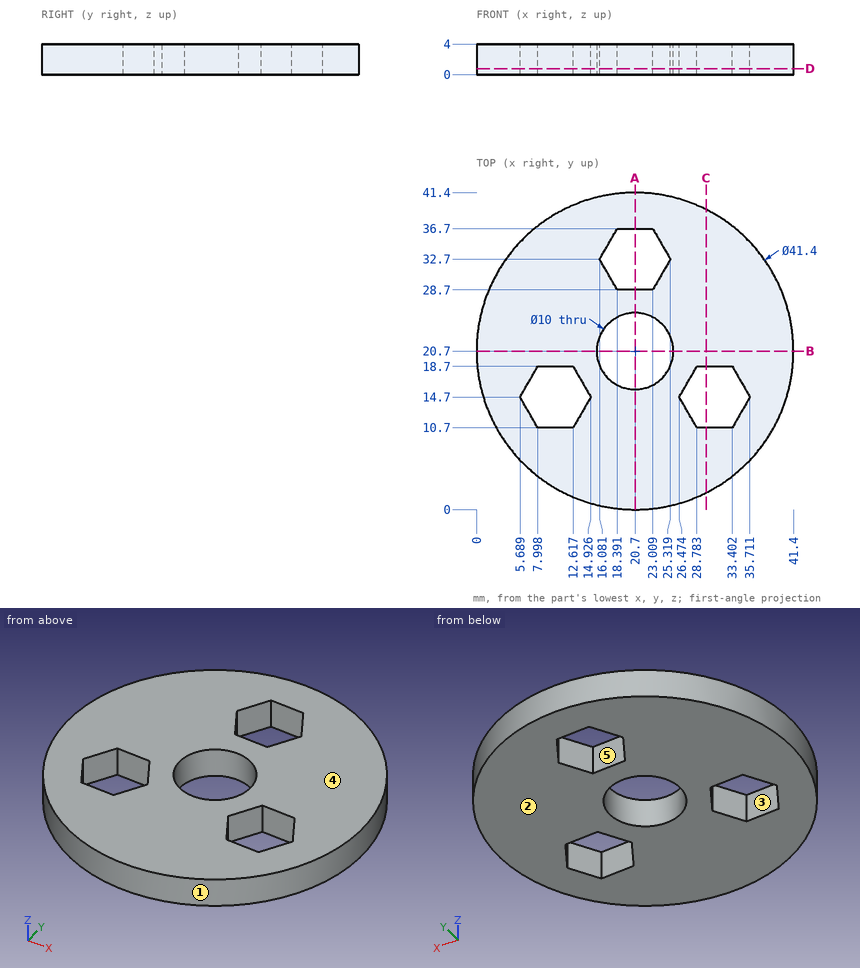
The drawing under review shows one solid part. Ordinate dimensions are in mm from its lowest x, y, z. A direction names the side the tool comes from. Coordinates: 2 decimals unless noted, no trailing zeros. Loops run counter-clockwise (first coordinate to the right, second up) from the corner with the lowest first, then second, coordinate; pieces in that order, holes last. Notation, with made-up numbers: (-36, 76) -> (4, 76) arc R13 cw to (4, 88) -> close; hole circle Ø11 at (24.5, 35). An arc over 180 degrees is marked (long way). Answer as a JSON object with one key per item and string values.
Q1. Take a section at B-B on y = 20.7. Give the boundary of the cut face in (x, z), plus the area to 3 significant figures.
Answer block:
{"outline": "(0, 0) -> (15.7, 0) -> (15.7, 4) -> (0, 4) -> close; (25.7, 0) -> (41.4, 0) -> (41.4, 4) -> (25.7, 4) -> close", "area": "126 mm^2"}
Q2. The part is to be moulded in two halves that separate along X. For the marked faces 1, 2 and 3, say which applies: +X half, -X half, draft (parallel to the pull), parting line (faces both ways), or undercut.
Answer block:
{"face 1": "parting line", "face 2": "draft", "face 3": "undercut"}
Q3. Tool access review of the marked faces 4 and 5: name each direction out of +Z, -Z, +X, -X, +Y, -Y from which nothing blocks a thin tool from reaching the whole face with its end or side.
Answer block:
{"face 4": "+Z, +X, -X, +Y, -Y", "face 5": "+Z, -Z"}
Q4. Take a section at A-A on x = 20.7. Give the boundary of the cut face in (y, z).
Answer block:
{"outline": "(0, 0) -> (15.7, 0) -> (15.7, 4) -> (0, 4) -> close; (25.7, 0) -> (28.7, 0) -> (28.7, 4) -> (25.7, 4) -> close; (36.7, 0) -> (41.4, 0) -> (41.4, 4) -> (36.7, 4) -> close"}
Q5. Clearance check with flat-ended pins moving along their axes: pin 1 Ø9 at (x, y) = (20.7, 20.7) entering from +Z; pin 2 Ø1 at (y, z) = (14.5, 2) entering from -X; pin 3 Ø1.5 at (y, z) = (14.5, 3.5) entering from +X; pin 4 Ø2 at (x, z) = (19.5, 2.5) entering from +Y. State where each tip first meets the part, or that it passes through.
Answer block:
{"pin 1": "passes through", "pin 2": "stops at x = 0.8", "pin 3": "stops at x = 40.67", "pin 4": "stops at y = 41.4"}
Q6. To check wall thickness, follow L1, parallel to Y at x = 20.7, z = 2.9; L2, parallel to X at y = 11, z = 0.65 (1 decimal); L3, parallel to Y at x = 23, z = 0.3 (1 decimal). State the ranges of each line that lie inside material, in increasing order.
Answer block:
{"L1": "y = 0 to 15.7, 25.7 to 28.7, 36.7 to 41.4", "L2": "x = 2.4 to 7.8, 12.8 to 28.6, 33.6 to 39", "L3": "y = 0.1 to 16.3, 25.1 to 28.7, 36.7 to 41.3"}
Q7. Take a section at D-D on z = 0.8. Give the boundary of the cut face in (x, y), plus the area to 3 significant figures.
Answer block:
{"outline": "circle Ø41.4 at (20.7, 20.7); hole (5.69, 14.7) -> (8, 10.7) -> (12.62, 10.7) -> (14.93, 14.7) -> (12.62, 18.7) -> (8, 18.7) -> close; hole circle Ø10 at (20.7, 20.7); hole (16.08, 32.7) -> (18.39, 28.7) -> (23.01, 28.7) -> (25.32, 32.7) -> (23.01, 36.7) -> (18.39, 36.7) -> close; hole (26.47, 14.7) -> (28.78, 10.7) -> (33.4, 10.7) -> (35.71, 14.7) -> (33.4, 18.7) -> (28.78, 18.7) -> close", "area": "1,100 mm^2"}
Q8. Take a section at C-C on x = 30. Give the boundary of the cut face in (y, z), plus the area to 3 significant figures.
Answer block:
{"outline": "(2.21, 0) -> (10.7, 0) -> (10.7, 4) -> (2.21, 4) -> close; (18.7, 0) -> (39.19, 0) -> (39.19, 4) -> (18.7, 4) -> close", "area": "116 mm^2"}
